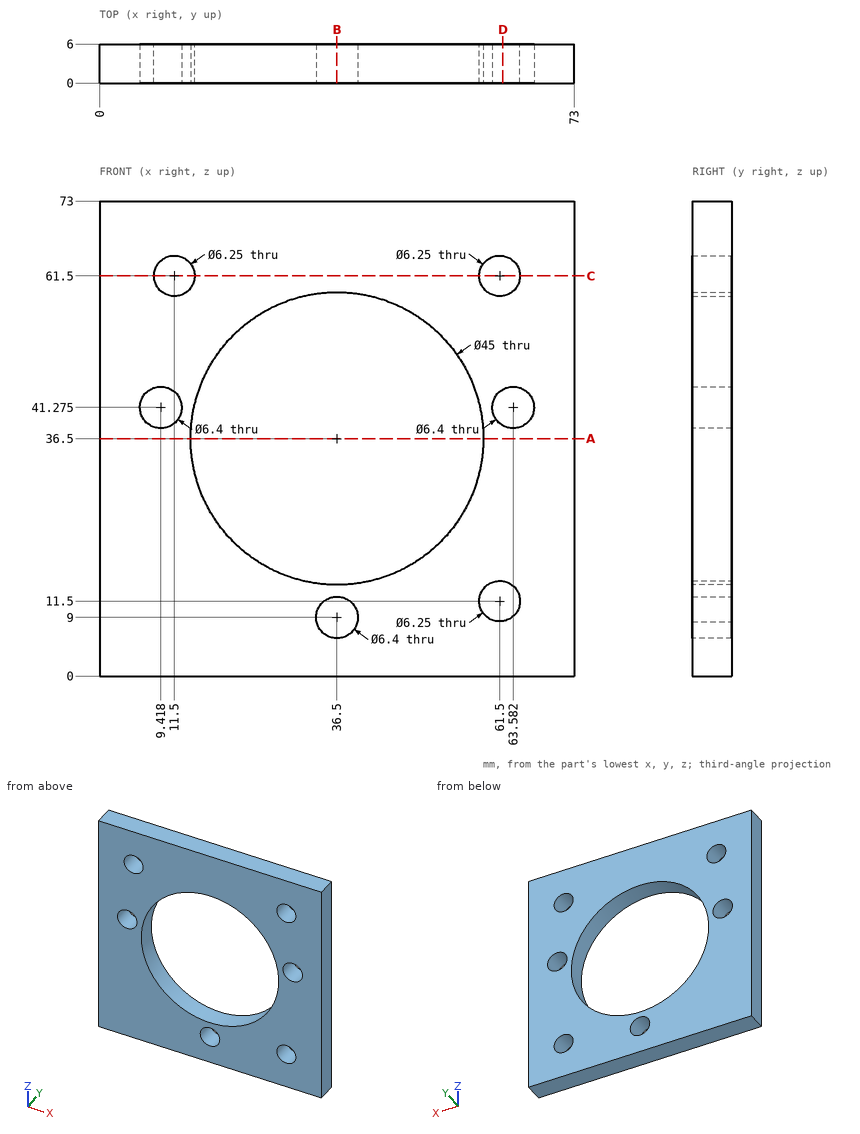
The drawing under review shows one solid part. Ordinate dimensions are in mm from its lowest x, y, z. Give positions to 0.01 mm unless a question says otherwise; leave off trailing zeros. Write each loop counter-clockwise with the first axis right and the second up, starting at its lowest first coordinate (ties: lowest second). Pieces come first, ordered by that corner, then holes. Notation, with made-up numbers: M 58.25,-35.75 L 62.25,-35.75 A20 ccw 62.25,1.25 Z; hole C 18.25,-40 d6. An arc over 180 degrees is marked long. Write each question's results on one line, items separated by ' | '. Start each with the question number.
1. We need section D-D (x = 62). Write out the cut boundary in (y, z) (1 decimal).
2. We need section C-C (z = 61.5). Write out the cut boundary in (x, y) (1 decimal).
3. We need section A-A (z = 36.5). Write out the cut boundary in (x, y).
4. We need section B-B (x = 36.5). Write out the cut boundary in (y, z).
5. For probe 1 along X at (y, z) = (4.5, 61.5) (1 decimal); probe 2 along X at (y, z) = (3.1, 36.5); probe 3 along X at (y, z) = (3.1, 10), list the stretches that pass through material, from the lowest coordinate up. Write a range as [from, to].
6. Insertion check: pin 1 Ø5 at (x, z) = (63.58, 41.28) entering from +Y. The pin has a flat end and moves straight along its axis. Give the tip position at first contact, or say it passes through.
Results found:
1) outline: M 0,0 L 6,0 L 6,8.4 L 0,8.4 Z; M 0,14.6 L 6,14.6 L 6,38.5 L 0,38.5 Z; M 0,44.1 L 6,44.1 L 6,58.4 L 0,58.4 Z; M 0,64.6 L 6,64.6 L 6,73 L 0,73 Z
2) outline: M 0,0 L 8.4,0 L 8.4,6 L 0,6 Z; M 14.6,0 L 58.4,0 L 58.4,6 L 14.6,6 Z; M 64.6,0 L 73,0 L 73,6 L 64.6,6 Z
3) outline: M 0,0 L 14,0 L 14,6 L 0,6 Z; M 59,0 L 73,0 L 73,6 L 59,6 Z
4) outline: M 0,0 L 6,0 L 6,5.8 L 0,5.8 Z; M 0,12.2 L 6,12.2 L 6,14 L 0,14 Z; M 0,59 L 6,59 L 6,73 L 0,73 Z
5) probe 1: x = [0, 8.4], [14.6, 58.4], [64.6, 73] | probe 2: x = [0, 14], [59, 73] | probe 3: x = [0, 33.46], [39.54, 58.76], [64.24, 73]
6) pin 1: passes through
